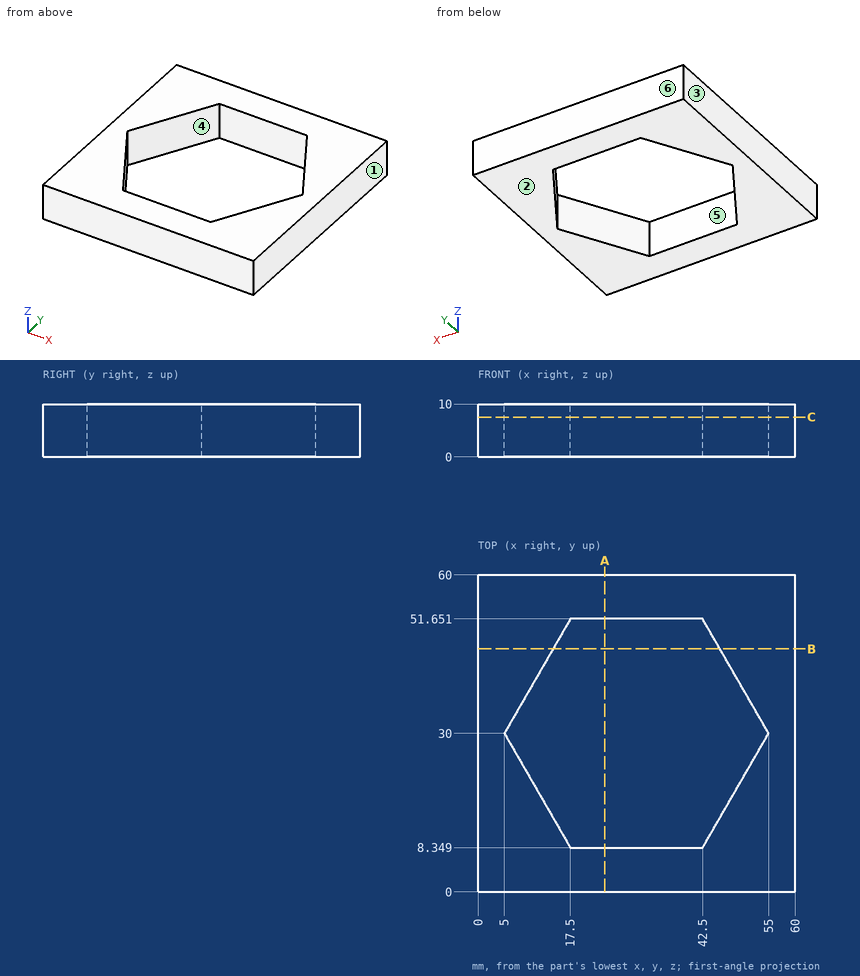
Verification items for this drawing (mm, ordinates from the low corner). A direction names the side the tool comes from. Give positions to 0.01 mm unless a question says otherwise; leave off trailing zeros. Loops run counter-clockwise (first coordinate to the right, second up) from the corner with the lowest first, then second, coordinate; pieces in that order, holes last. Notation, with made-up numbers: M 11.5,25.5 L 39.5,25.5 A22 ccw 39.5,35.5 Z; hole C 85,24 d11. An arc over 180 degrees is marked long. Answer as a JSON object with one key per item and string values. Group by question number.
Item 1: Material ranges on L1, parallel to Y at x = 36, z = 2.75; L2, parallel to Y at x = 47.5, z = 2.5; L3, parallel to X at y = 49, z = 1, recorded low to high.
Item 2: Sectioned sample at A-A on x = 24. Record the boundary of the cut face in (y, z), plus the area to 3 significant figures.
Item 3: Sectioned sample at B-B on y = 46. Record the boundary of the cut face in (x, z), plus the area to 3 significant figures.
Item 4: Mould release check, pull along X, two halves, no side actions. Record for the marked faces 1, 2, 3 and 4: pulls with the +X half, pulls with the -X half, needs draft (parallel to the pull), parting line crosses it, or undercut.
Item 5: Sectioned sample at C-C on z = 7.5. Record the boundary of the cut face in (x, y), plus the area to 3 significant figures.
Item 6: Access from +Z, -Z, +X, -X, +Y, -Y to the whole of each face (thin tool, end or side, straight path). Record for the marked faces 5 and 6.
Findings below:
{
 "1": {"L1": "0 to 8.35, 51.65 to 60", "L2": "0 to 17.01, 42.99 to 60", "L3": "0 to 15.97, 44.03 to 60"},
 "2": {"outline": "M 0,0 L 8.35,0 L 8.35,10 L 0,10 Z; M 51.65,0 L 60,0 L 60,10 L 51.65,10 Z", "area": "167 mm2"},
 "3": {"outline": "M 0,0 L 14.24,0 L 14.24,10 L 0,10 Z; M 45.76,0 L 60,0 L 60,10 L 45.76,10 Z", "area": "285 mm2"},
 "4": {"face 1": "pulls with the +X half", "face 2": "needs draft", "face 3": "pulls with the -X half", "face 4": "undercut"},
 "5": {"outline": "M 0,0 L 60,0 L 60,60 L 0,60 Z; hole M 5,30 L 17.5,8.35 L 42.5,8.35 L 55,30 L 42.5,51.65 L 17.5,51.65 Z", "area": "1,980 mm2"},
 "6": {"face 5": "+Z, -Z", "face 6": "+Z, -Z, +X, -X, +Y"}
}
